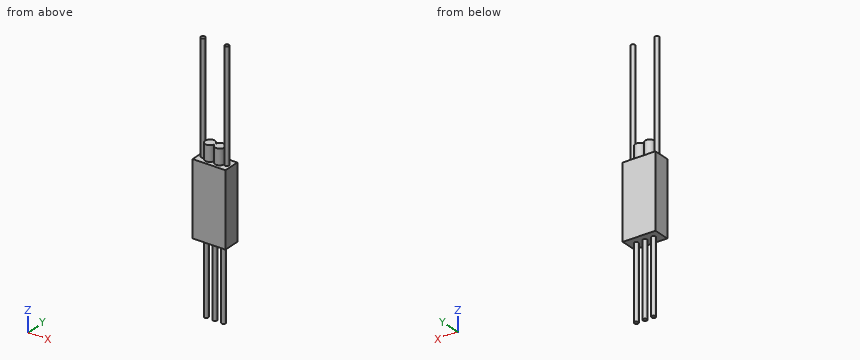
Autodesk Inventor part; units mm, degrees
ref_plane "YZ Plane" through (0, 0, 0) normal (1, 0, 0) x (0, 1, 0)
ref_plane "XZ Plane" through (0, 0, 0) normal (0, 1, 0) x (-1, 0, 0)
ref_plane "XY Plane" through (0, 0, 0) normal (0, 0, 1) x (1, 0, 0)
sketch "Sketch1" plane through (0, 0, 0) normal (0, 1, 0) x (-1, 0, 0)
  line L0 (17, 38) -> (-17, 38)
  line L1 (-17, 38) -> (-17, -38)
  line L2 (-17, -38) -> (17, -38)
  line L3 (17, -38) -> (17, 38)
  line L4 (23.8, 0) -> (-23.8, 0)
  line L5 (0, -53.2) -> (0, 53.2)
  point P0 (0, 0)
  dimension "d0" = 76
  dimension "d1" = 34
extrude "Extrusion1" add sketch "Sketch1" along normal mid plane 17
sketch "Sketch2" plane through (-17, 8.5, 38) normal (0, 0, 1) x (1, 0, 0)
  line L0 (34, -17) -> (34, 0)
  line L1 (0, 0) -> (34, 0)
  line L2 (0, 0) -> (0, -17)
  line L3 (34, -17) -> (0, -17)
  circle A0 centre (11.85, -8.5) radius 5.15
  circle A1 centre (22.15, -8.5) radius 5.15
  line L4 (11.85, -8.5) -> (22.15, -8.5) construction
  circle A2 centre (4.55, -8.5) radius 2.15
  circle A3 centre (29.45, -8.5) radius 2.15
  point P0 (17, -8.5)
  point P1 (17, -8.5)
  dimension "d4" = 10.3
  dimension "d7" = 4.3
extrude "Extrusion2" add sketch "Sketch2" along normal blind 16 contours A0 | A1
extrude "Extrusion3" add sketch "Sketch2" along normal blind 114.3 contours A2 | A3
sketch "Sketch3" plane through (17, 8.5, -38) normal (0, 0, -1) x (-1, 0, 0)
  circle A0 centre (17, -8.5) radius 2.15
  circle A1 centre (26, -8.5) radius 2.15
  circle A2 centre (8, -8.5) radius 2.15
  dimension "d10" = 4.3
  dimension "d11" = 9
  dimension "d12" = 9
extrude "Extrusion4" add sketch "Sketch3" along normal blind 76.2
properties part number "Turnigy_ESC" material "PPS Plastic"
Verification items for the finished model (mm, model axes). Round coordinates to 2 decimals unless told otherwise and drop trailing zeros. Loops run counter-clockwise (first coordinate to the right, second up) from the corner with the lowest first, then second, coordinate; pieces in that order, holes last. Notation, with made-up numbers: (64.25, 48) - (115.25, 48) arc R30 cw to (115.25, 80) - close; hole circle Ø1 at (29.5, 33.25). An arc over 180 degrees is marked (long way). Answer in a Markdown table with one row per item. Add a question column.
Q1. Section check B-B on z = 71.5. Enter the section's corners in (x, y).
Q2. Gauge pin test, flat ends, axial feed: pin 1 (10 mm diameter, centred on y = -6.5, z = -75, fed in from -X); pin 2 (5 mm diameter, centred on x = 7, y = 1, fed in from +Z); pin 3 (3 mm diameter, centred on y = -1.5, z = -80.5, fed in from +X). Record the tip position at first contact, or that the pin passes through.
Q3. Section check A-A on z = -87. Enter the section's corners in (x, y), plus the area to 3 significant figures.
Q4. Material ranges on line 1 (Y direction, x = -9, z = -81); line 2 (Z direction, x = -7.5, y = 6.25); line 3 (Z direction, x = -3, y = 2.25), recorded low to high.
Found:
| question | item | result |
|---|---|---|
| 1 | outline | circle Ø4.3 at (-12.45, 0); circle Ø4.3 at (12.45, 0) |
| 2 | pin 1 | stops at x = -10.54 |
| 2 | pin 2 | stops at z = 54 |
| 2 | pin 3 | stops at x = 11.15 |
| 3 | outline | circle Ø4.3 at (-9, 0); circle Ø4.3 at (0, 0); circle Ø4.3 at (9, 0) |
| 3 | area | 43.6 mm² |
| 4 | line 1 | y = -2.15 to 2.15 |
| 4 | line 2 | z = -38 to 38 |
| 4 | line 3 | z = -38 to 54 |
